Autodesk Inventor part; units mm, degrees
ref_plane "YZ Plane" through (0, 0, 0) normal (1, 0, 0) x (0, 1, 0)
ref_plane "XZ Plane" through (0, 0, 0) normal (0, 1, 0) x (-1, 0, 0)
ref_plane "XY Plane" through (0, 0, 0) normal (0, 0, 1) x (1, 0, 0)
sketch "Sketch1" plane through (0, 0, 0) normal (1, 0, 0) x (0, 1, 0)
  circle A0 centre (0, 0) radius 10.5
  dimension "d0" = 21
extrude "Extrusion1" add sketch "Sketch1" along normal blind 222
sketch "Sketch2" plane through (222, 0, 0) normal (1, 0, 0) x (0, 0, -1)
  circle A0 centre (0, 0) radius 3
  dimension "d3" = 6
extrude "Extrusion2" add sketch "Sketch2" along normal blind 22
sketch "Sketch3" plane through (0, 0, 0) normal (-1, 0, 0) x (0, 0, 1)
  circle A0 centre (0, 0) radius 3
  dimension "d6" = 6
extrude "Extrusion3" add sketch "Sketch3" along normal blind 15
sketch "Sketch4" plane through (-15, 0, 0) normal (-1, 0, 0) x (0, 0, 1)
  circle A0 centre (0, 0) radius 2
  dimension "d9" = 4
extrude "Extrusion4" add sketch "Sketch4" along normal blind 4
sketch "Sketch5" plane through (-19, 0, 0) normal (-1, 0, 0) x (0, 0, 1)
  circle A0 centre (0, 0) radius 3
  dimension "d12" = 6
extrude "Extrusion5" add sketch "Sketch5" along normal blind 2
properties part number "RouleauIdler"
Source: CAD feature listing. Evaluate the final solid. Frame: model axes, mm. A direction names the side the tool comes from. Coordinates: 2 decimals unless noted, no trailing zeros. Loops run counter-clockwise (first coordinate to the right, second up) from the corner with the lowest first, then second, coordinate; pieces in that order, holes last. Notation, with made-up numbers: (-36, 78) - (-29, 78) arc R21 ccw to (-29, 104) - close; hole circle Ø5 at (13, 76.5). An arc over 180 degrees is marked (long way). Answer as CSV lines item,"result".
1. Ray query, line 1 (X direction, y = 3.5, z = -7.25); line 2 (Z direction, x = 105.5, y = -1); line 3 (Y direction, x = 226, z = 0.25). Return the intervals inside material, ascending.
Established:
line 1,"x = 0 to 222"
line 2,"z = -10.45 to 10.45"
line 3,"y = -2.99 to 2.99"
2. Section A-A (x = 202). Return loops of the section in (y, z).
Established:
outline,"circle Ø21 at (0, 0)"
3. Section B-B (z = -5.25). Return loops of the section in (x, y), then the cut area to 3 significant figures.
Established:
outline,"(0, -9.09) - (222, -9.09) - (222, 9.09) - (0, 9.09) - close"
area,"4,040 mm2"
4. Mould query, pull axis X, two halves, no side actions, for faces 6 (the flat face through (-15, -2, 1)), 7 (the cylindrical face through (-17, 2, 0)), 8 (the flat face through (0, 2.2, 2.5)), 9 (the cylindrical face through (-7, 0, -3)). Classes: released by +X, released by -X, zero draft, split by the parting line, or undercut.
Established:
face 6,"undercut"
face 7,"undercut"
face 8,"released by -X"
face 9,"zero draft"
5. Section C-C (y = -7.5). Return loops of the section in (x, z), then the cut area to 3 significant figures.
Established:
outline,"(0, -7.35) - (222, -7.35) - (222, 7.35) - (0, 7.35) - close"
area,"3,260 mm2"
6. Reachability of faces 1 (the flat face through (244, 0, 0)), 2 (the flat face through (-21, 0, 0)), 3 (the cylindrical face through (233, 0, 3)), 4 (the flat face through (-19, -2, 1)), 5 (the cylindrical face through (-20, 0, -3)) from +Z, -Z, +X, -X, +Y, -Y: full face, straight path, thin tool, end or side. Return the list, or none.
Established:
face 1,"+Z, -Z, +X, +Y, -Y"
face 2,"+Z, -Z, -X, +Y, -Y"
face 3,"+X"
face 4,"none"
face 5,"-X"
7. Contact query for flat-ended pins moving along their axis: pin 1 (10 mm diameter, centred on x = 99.5, y = 6, fed in from -Z); pin 2 (10.5 mm diameter, centred on y = 2.5, z = -3, fed in from +X); pin 3 (12 mm diameter, centred on x = 143, z = 8, fed in from -Y); pin 4 (1.5 mm diameter, centred on x = 169, z = -3.5, fed in from +Y). Output: stop coordinate, or through.
Established:
pin 1,"stops at z = -10.45"
pin 2,"stops at x = 244"
pin 3,"stops at y = -10.31"
pin 4,"stops at y = 10.13"
